Here's how the part is built. I have some questions about the finished solid (model axes, mm). Coordinates: 2 decimals unless noted, no trailing zeros. Loops run counter-clockwise (first coordinate to the right, second up) from the corner with the lowest first, then second, coordinate; pieces in that order, holes last. Notation, with made-up numbers: (-7.5, 72.5) -> (16.5, 72.5) arc R28 cw to (16.5, 104.5) -> close; hole circle Ø1 at (57, 81). An arc over 180 degrees is marked (long way). Answer as a JSON object with one key per item and string values. Group by question number.
Q1. I'm going to push a flat-ended pin straight in: pin 1 (1.5 mm diameter, centred on x = 0.5, z = -56, fed in from +Y). Where does the tip first touch, or does it pass through?
Q2. I want a section at A-A on x = 2.2. Write out the boundary of the cut face in (y, z), then the cut area to 3 significant figures.
Q3. I want a section at B-B on z = -85. Write out the boundary of the cut face in (x, y).
Q4. I need wall thicknesses on line 1 (Y direction, x = 2.35, z = -87.5); line 2 (Y direction, x = 2.4, z = -14); line 3 (Z direction, x = 2.4, y = 9.5). Which ranges of each line are inside material? Lowest first, please.
Q5. I want a section at C-C on y = 13.25. Write out the boundary of the cut face in (x, z).
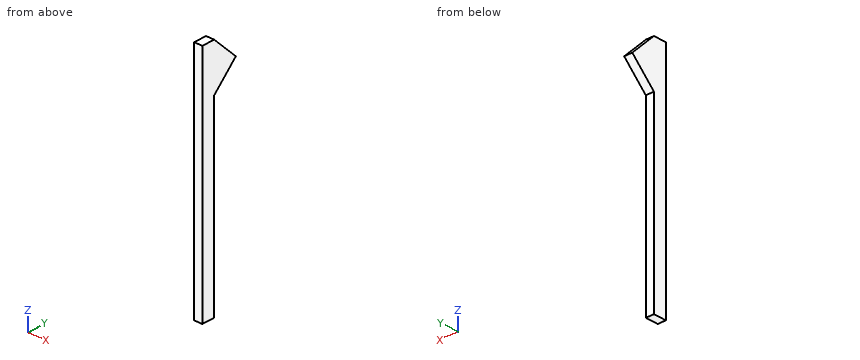
```python
from build123d import *

# Parameters (mm, degrees)
ESQUISSE1_W        = 3.5
ESQUISSE1_H        = 5.5
BOSS_EXTRU_1_DEPTH = 100
BOSS_EXTRU_2_DEPTH = 3.5


with BuildPart() as part:
    # Esquisse1 → Boss.-Extru.1 (new body)
    with BuildSketch(Plane.XY):
        with Locations((1.75, 2.75)):
            Rectangle(ESQUISSE1_W, ESQUISSE1_H)
    extrude(amount=-BOSS_EXTRU_1_DEPTH)

    # Esquisse2 → Boss.-Extru.2 (add)
    with BuildSketch(Plane.ZY):
        Polygon((0, 5.5), (-10, 5.5), (-20, 5.5), (-10, 15.5), align=None)
    extrude(amount=-BOSS_EXTRU_2_DEPTH)


solid = part.part
```
Result set:
{
 "1": {"pin 1": "stops at y = 5.5"},
 "2": {"outline": "(0, -100) -> (5.5, -100) -> (5.5, -20) -> (15.5, -10) -> (5.5, 0) -> (0, 0) -> close", "area": "650 mm²"},
 "3": {"outline": "(0, 0) -> (3.5, 0) -> (3.5, 5.5) -> (0, 5.5) -> close"},
 "4": {"line 1": "y = 0 to 5.5", "line 2": "y = 0 to 11.5", "line 3": "z = -16 to -4"},
 "5": {"outline": "(0, -12.25) -> (3.5, -12.25) -> (3.5, -7.75) -> (0, -7.75) -> close"}
}
